Could you check a few things on this model? Use its own coordinates, in mm. Face numbers are marked on the shaded views. A direction names the side the tool comes from. Coordinates: 2 decimals unless noted, no trailing zeros.
Item 1: If I drill on probe 1 along X at (y, z) = (11, -44); probe 2 along Z at (x, y) = (74.5, 14.25); probe 3 along Z at (x, y) = (-83, 5.25), over which ranges is the centre line in solid material (lowest first)?
Item 2: Thinking about a two-plate mould opening in X: for the marked faces 5, 6, 7 and 8, which applies, +X half, -X half, draft (parallel to the pull), parting line (faces both ways), or undercut?
Item 3: For P1, Ø12, axis at x = 64, y = 21, coming from the +Z side; P2, Ø1, axis at x = 34, z = -39, coming from the -Y side; P3, Ø5, axis at x = -65.5, y = 13.5, coming from the -Z side, each with a flat end and sliding along its axis, tell me the tip position at first contact or that it passes through.
Item 4: I want a section at A-A on y = 11.25. State how many separate pieces and enclosed holes the cut face has, then the cut area to 3 significant figures.
Item 5: Which directions (+Z, -Z, +X, -X, +Y, -Y) give clear straight access to the entire face, cutting with the end or side of a thin tool? Please do the marked faces 1, 2, 3 and 4.
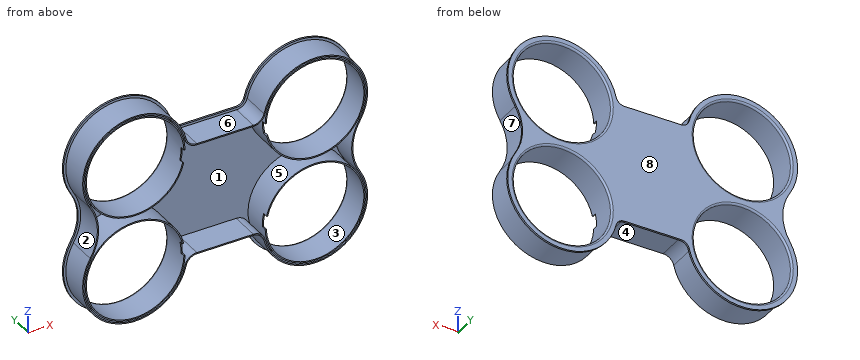
from build123d import *

# Parameters (mm, degrees)
SKETCH1_R           = 40.4
BOSS_EXTRUDE1_DEPTH = 25
SHELL1_T            = -1
FILLET1_R           = 1.5
SWEEP3_START        = 23.5
SWEEP3_DEPTH        = 1.5
CUT_EXTRUDE1_DEPTH  = 4


# Read off the part's stored shape, not the designer's step: Sweep3
with BuildPart() as part:
    # Sketch1 → Boss-Extrude1 (new body)
    with BuildSketch(Plane(origin=(0, 0, 0), x_dir=(1, 0, 0), z_dir=(0, 1, 0))):
        with BuildLine():
            Line((-23.389824888, -47), (23.389824888, -47))
            ThreePointArc((23.389824888, -47), (28.979355918, -48.946125685), (32.151569193, -53.942857143))
            ThreePointArc((32.151569193, -53.942857143), (90.931692418, -84.277158344), (111.718349922, -21.482352941))
            ThreePointArc((111.718349922, -21.482352941), (105.725511342, 0), (111.718349922, 21.482352941))
            ThreePointArc((111.718349922, 21.482352941), (90.931692418, 84.277158344), (32.151569193, 53.942857143))
            ThreePointArc((32.151569193, 53.942857143), (28.979355918, 48.946125685), (23.389824888, 47))
            Line((23.389824888, 47), (-23.389824888, 47))
            ThreePointArc((-23.389824888, 47), (-28.979355918, 48.946125685), (-32.151569193, 53.942857143))
            ThreePointArc((-32.151569193, 53.942857143), (-90.931692418, 84.277158344), (-111.718349922, 21.482352941))
            ThreePointArc((-111.718349922, 21.482352941), (-105.725511342, 0), (-111.718349922, -21.482352941))
            ThreePointArc((-111.718349922, -21.482352941), (-90.931692418, -84.277158344), (-32.151569193, -53.942857143))
            ThreePointArc((-32.151569193, -53.942857143), (-28.979355918, -48.946125685), (-23.389824888, -47))
        make_face()
        with Locations(Location((74.5, -44, 0), (0, 0, 270))):
            Circle(SKETCH1_R, mode=Mode.SUBTRACT)
        with Locations(Location((74.5, 44, 0), (0, 0, 270))):
            Circle(SKETCH1_R, mode=Mode.SUBTRACT)
        with Locations(Location((-74.5, 44, 0), (0, 0, 270))):
            Circle(SKETCH1_R, mode=Mode.SUBTRACT)
        with Locations(Location((-74.5, -44, 0), (0, 0, 270))):
            Circle(SKETCH1_R, mode=Mode.SUBTRACT)
    extrude(amount=BOSS_EXTRUDE1_DEPTH)

    # Shell1
    shell1_openings = [part.faces().sort_by_distance(p)[0] for p in [
        (0, 0, 0),
    ]]
    offset(amount=SHELL1_T, openings=shell1_openings, kind=Kind.INTERSECTION)

    # Fillet1
    fillet1_edges = [part.edges().sort_by_distance(p)[0] for p in [
        (74.5, 25, 3.6),
        (74.5, 25, -84.4),
        (-74.5, 25, -84.4),
        (-74.5, 25, 3.6),
    ]]
    fillet(fillet1_edges, radius=FILLET1_R)

    # Sweep3 outline → Sweep3 (add)
    with BuildSketch(Plane(origin=(0, 0, 0), x_dir=(1, 0, 0), z_dir=(0, 1, 0)).offset(SWEEP3_START)):
        with BuildLine():
            Line((-23.389824888, -49), (23.389824888, -49))
            ThreePointArc((23.389824888, -49), (27.737237912, -50.51365331), (30.204514903, -54.4))
            ThreePointArc((30.204514903, -54.4), (91.687172529, -86.128981716), (113.429538424, -20.447058824))
            ThreePointArc((113.429538424, -20.447058824), (107.725511342, 0), (113.429538424, 20.447058824))
            ThreePointArc((113.429538424, 20.447058824), (91.687172529, 86.128981716), (30.204514903, 54.4))
            ThreePointArc((30.204514903, 54.4), (27.737237912, 50.51365331), (23.389824888, 49))
            Line((23.389824888, 49), (-23.389824888, 49))
            ThreePointArc((-23.389824888, 49), (-27.737237912, 50.51365331), (-30.204514903, 54.4))
            ThreePointArc((-30.204514903, 54.4), (-91.687172529, 86.128981716), (-113.429538424, 20.447058824))
            ThreePointArc((-113.429538424, 20.447058824), (-107.725511342, 0), (-113.429538424, -20.447058824))
            ThreePointArc((-113.429538424, -20.447058824), (-91.687172529, -86.128981716), (-30.204514903, -54.4))
            ThreePointArc((-30.204514903, -54.4), (-27.737237912, -50.51365331), (-23.389824888, -49))
        make_face()
        with BuildLine():
            ThreePointArc((-111.718349922, -21.482352941), (-105.725511342, 0), (-111.718349922, 21.482352941))
            ThreePointArc((-111.718349922, 21.482352941), (-90.931692418, 84.277158344), (-32.151569193, 53.942857143))
            ThreePointArc((-32.151569193, 53.942857143), (-28.979355918, 48.946125685), (-23.389824888, 47))
            Line((-23.389824888, 47), (23.389824888, 47))
            ThreePointArc((23.389824888, 47), (28.979355918, 48.946125685), (32.151569193, 53.942857143))
            ThreePointArc((32.151569193, 53.942857143), (90.931692418, 84.277158344), (111.718349922, 21.482352941))
            ThreePointArc((111.718349922, 21.482352941), (105.725511342, 0), (111.718349922, -21.482352941))
            ThreePointArc((111.718349922, -21.482352941), (90.931692418, -84.277158344), (32.151569193, -53.942857143))
            ThreePointArc((32.151569193, -53.942857143), (28.979355918, -48.946125685), (23.389824888, -47))
            Line((23.389824888, -47), (-23.389824888, -47))
            ThreePointArc((-23.389824888, -47), (-28.979355918, -48.946125685), (-32.151569193, -53.942857143))
            ThreePointArc((-32.151569193, -53.942857143), (-90.931692418, -84.277158344), (-111.718349922, -21.482352941))
        make_face(mode=Mode.SUBTRACT)
    extrude(amount=SWEEP3_DEPTH)

    # Sketch11 → Cut-Extrude1 (cut)
    with BuildSketch(Plane(origin=(0, 0, 0), x_dir=(1, 0, 0), z_dir=(0, 1, 0))):
        with BuildLine():
            Line((-33.218669872, 45.046086874), (-34.11587702, 45.132524243))
            ThreePointArc((-34.11587702, 45.132524243), (-34.304886561, 39.936398688), (-35.15969651, 34.807583489))
            ThreePointArc((-35.15969651, 34.807583489), (-34.700986823, 34.532231781), (-34.274323948, 34.20944403))
            ThreePointArc((-34.274323948, 34.20944403), (-33.336128547, 39.584607949), (-33.112976312, 45.036470093))
            ThreePointArc((-33.112976312, 45.036470093), (-33.16583585, 45.041138266), (-33.218669872, 45.046086874))
        make_face()
        with BuildLine():
            ThreePointArc((33.218669872, 45.046086874), (33.16583585, 45.041138266), (33.112976312, 45.036470093))
            ThreePointArc((33.112976312, 45.036470093), (33.336128547, 39.584607949), (34.274323948, 34.20944403))
            ThreePointArc((34.274323948, 34.20944403), (34.700986823, 34.532231781), (35.15969651, 34.807583489))
            ThreePointArc((35.15969651, 34.807583489), (34.304886561, 39.936398688), (34.11587702, 45.132524243))
            Line((34.11587702, 45.132524243), (33.218669872, 45.046086874))
        make_face()
        with BuildLine():
            ThreePointArc((-33.112976312, -45.036470093), (-33.336128547, -39.584607949), (-34.274323948, -34.20944403))
            ThreePointArc((-34.274323948, -34.20944403), (-34.700986823, -34.532231781), (-35.15969651, -34.807583489))
            ThreePointArc((-35.15969651, -34.807583489), (-34.304886561, -39.936398688), (-34.11587702, -45.132524243))
            Line((-34.11587702, -45.132524243), (-33.218669872, -45.046086874))
            ThreePointArc((-33.218669872, -45.046086874), (-33.16583585, -45.041138266), (-33.112976312, -45.036470093))
        make_face()
        with BuildLine():
            ThreePointArc((35.15969651, -34.807583489), (34.700986823, -34.532231781), (34.274323948, -34.20944403))
            ThreePointArc((34.274323948, -34.20944403), (33.336128547, -39.584607949), (33.112976312, -45.036470093))
            ThreePointArc((33.112976312, -45.036470093), (33.16583585, -45.041138266), (33.218669872, -45.046086874))
            Line((33.218669872, -45.046086874), (34.11587702, -45.132524243))
            ThreePointArc((34.11587702, -45.132524243), (34.304886561, -39.936398688), (35.15969651, -34.807583489))
        make_face()
    extrude(amount=CUT_EXTRUDE1_DEPTH, mode=Mode.SUBTRACT)


solid = part.part
Response values:
1. probe 1: x = -118 to -117, -115.9 to -114.9, -34.1 to -33.1, 33.1 to 34.1, 114.9 to 115.9, 117 to 118
1. probe 2: z = -87.5 to -86.5, -85.4 to -84.4, -3.6 to -2.6, 2.6 to 3.6, 84.4 to 85.4, 86.5 to 87.5
1. probe 3: z = -86.66 to -85.64, -84.52 to -83.5, -4.5 to -3.48, 3.48 to 4.5, 83.5 to 84.52, 85.64 to 86.66
2. face 5: undercut
2. face 6: undercut
2. face 7: +X half
2. face 8: draft
3. P1: stops at z = 89.22
3. P2: stops at y = 4
3. P3: stops at z = -87.01
4. separate pieces: 5
4. enclosed holes: 5
4. area: 1,860 mm2
5. face 1: -Y
5. face 2: -X, -Y
5. face 3: +Y, -Y
5. face 4: -Z, -Y
